Here's how the part is built. I have some questions about the finished solid (model axes, mm). Face numbers are marked on the shaded views. Coordinates: 2 decimals unless noted, no trailing zeros. Write each loop counter-clockwise with the first axis right and the second up, starting at its lowest first coordinate (ties: lowest second). Pieces come first, ordered by that corner, then holes.
(1) Imagine slicing it at C-C, the plane z = 0.75. List the corners of the cut face in (x, y) for me.
(2) Thinking about a two-plate mould opening in Y: for the marked faces 1, 2, 3 and 4, which applies, released by +Y, released by -Y, zero draft, split by the parting line, or undercut?
(3) Imagine slicing it at A-A, the plane y = -6.6. List the corners of the cut face in (x, z) for me, plus the area to 3 significant figures.
(4) For pin 1 Ø2.5 at (y, z) = (-11, 3) entering from -X; pin 2 Ø0.5 at (x, y) = (-6.5, 1) entering from -Z; pin 3 Ø3 at (x, z) = (-5, 5.5) entering from -Y, each with a flat end and sliding along its axis, tell me the tip position at first contact or that it passes through.
(5) Imagine slicing it at B-B, the plane x = 3. List the corners of the cut face in (y, z) for me.
(6) Please list where these lines run through material, in increasing order: probe 1 along X at (y, z) = (-6.5, 4); probe 2 along X at (y, z) = (-10.25, 4.25); probe 3 along Y at (x, z) = (-4.25, 4.25).
(7) Imagine slicing it at D-D, the plane y = -11.5. List the corners of the cut face in (x, z) for me, plus the area to 3 significant figures.
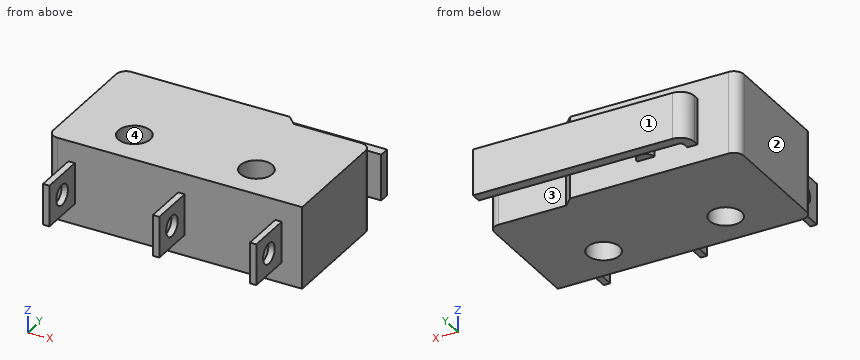
```python
from build123d import *

# Parameters (mm, degrees)
F0_W     = 0.5
F0_H     = 3.5
F0_R     = 1.25
F1_DEPTH = 6.4
F2_W     = 1.5
F2_H     = 1.4
F2_W_2   = 3.5
F2_H_2   = 1.6
F2_R     = 0.8
F3_DEPTH = 19.8
F4_R     = 0.762


with BuildPart() as f1:
    # F0 (on Top) → F1 (new body)
    with BuildSketch(Plane.XY):
        with Locations((4.1668843009, -11.25)):
            Rectangle(F0_W, F0_H)
        with Locations((-3.3831156991, -11.25)):
            Rectangle(F0_W, F0_H)
        with Locations((-11.9331156991, -11.25)):
            Rectangle(F0_W, F0_H)
        with BuildLine():
            Line((-10.6081156991, 0.7), (-9.8143656991, 0.7))
            Line((-9.8143656991, 0.7), (-9.8143656991, 1.101979753))
            ThreePointArc((-9.8143656991, 1.101979753), (-9.7252470071, 1.317131308), (-9.5100954521, 1.40625))
            Line((-9.5100954521, 1.40625), (6.0168843009, 1.40625))
            Line((6.0168843009, 1.40625), (6.0168843009, 2.2))
            Line((6.0168843009, 2.2), (-9.5100954521, 2.2))
            ThreePointArc((-9.5100954521, 2.2), (-10.2865130147, 1.8783973155), (-10.6081156991, 1.101979753))
            Line((-10.6081156991, 1.101979753), (-10.6081156991, 0.7))
        make_face()
        with BuildLine():
            Line((6.0168843009, 0), (0, 0))
            Line((0, 0), (-0.7, 0.7))
            Line((-0.7, 0.7), (-5.9126656991, 0.7))
            ThreePointArc((-5.9126656991, 0.7), (-6.5935156991, 1.38085), (-7.2743656991, 0.7))
            Line((-7.2743656991, 0.7), (-9.8143656991, 0.7))
            Line((-9.8143656991, 0.7), (-10.6081156991, 0.7))
            Line((-10.6081156991, 0.7), (-13.7831156991, 0.7))
            Line((-13.7831156991, 0.7), (-13.7831156991, -9.5))
            Line((-13.7831156991, -9.5), (-12.1831156991, -9.5))
            Line((-12.1831156991, -9.5), (-11.6831156991, -9.5))
            Line((-11.6831156991, -9.5), (-3.6331156991, -9.5))
            Line((-3.6331156991, -9.5), (-3.1331156991, -9.5))
            Line((-3.1331156991, -9.5), (3.9168843009, -9.5))
            Line((3.9168843009, -9.5), (4.4168843009, -9.5))
            Line((4.4168843009, -9.5), (6.0168843009, -9.5))
            Line((6.0168843009, -9.5), (6.0168843009, 0))
        make_face()
        with Locations((-8.6831156991, -6.6)):
            Circle(F0_R, mode=Mode.SUBTRACT)
        with Locations((0.8168843009, -6.6)):
            Circle(F0_R, mode=Mode.SUBTRACT)
    extrude(amount=F1_DEPTH)

    # F2 (on face) → F3 (cut, through all)
    with BuildSketch(Plane(origin=(-13.7831156991, 0, 0), x_dir=(0, -1, 0), z_dir=(-1, 0, 0))):
        with Locations((-1.45, 0.7)):
            Rectangle(F2_W, F2_H)
        with Locations((-1.45, 5.7)):
            Rectangle(F2_W, F2_H)
        with Locations((11.25, 0.8)):
            Rectangle(F2_W_2, F2_H_2)
        with Locations((11.25, 5.6)):
            Rectangle(F2_W_2, F2_H_2)
        with Locations((11.25, 3.2)):
            Circle(F2_R)
    extrude(amount=-F3_DEPTH, mode=Mode.SUBTRACT)

    # F4
    f4_edges = [f1.edges().sort_by_distance(p)[0] for p in [
        (-13.783116, -9.5, 3.2),
        (6.016884, 0, 3.2),
        (-13.783116, 0.7, 3.2),
    ]]
    fillet(f4_edges, radius=F4_R)


solid = f1.part
```
Recorded:
1. outline: (-13.78, -8.74) arc R0.76 ccw to (-13.02, -9.5) - (6.02, -9.5) - (6.02, -0.76) arc R0.76 ccw to (5.25, 0) - (0, 0) - (-0.7, 0.7) - (-13.02, 0.7) arc R0.76 ccw to (-13.78, -0.06) - close; hole circle Ø2.5 at (-8.68, -6.6); hole circle Ø2.5 at (0.82, -6.6)
2. face 1: released by +Y
2. face 2: zero draft
2. face 3: undercut
2. face 4: undercut
3. outline: (-13.78, 0) - (-9.93, 0) - (-9.93, 6.4) - (-13.78, 6.4) - close; (-7.43, 0) - (-0.43, 0) - (-0.43, 6.4) - (-7.43, 6.4) - close; (2.07, 0) - (6.02, 0) - (6.02, 6.4) - (2.07, 6.4) - close
3. area: 94.7 mm2
4. pin 1: stops at x = -12.18
4. pin 2: stops at z = 1.4
4. pin 3: stops at y = -9.5
5. outline: (-9.5, 0) - (0, 0) - (0, 6.4) - (-9.5, 6.4) - close; (1.41, 1.4) - (2.2, 1.4) - (2.2, 5) - (1.41, 5) - close
6. probe 1: x = -13.78 to -9.93, -7.44 to -0.43, 2.06 to 6.02
6. probe 2: x = -12.18 to -11.68, -3.63 to -3.13, 3.92 to 4.42
6. probe 3: y = -9.5 to 0.7, 1.41 to 2.2
7. outline: (-12.18, 1.6) - (-11.68, 1.6) - (-11.68, 2.44) - (-12.18, 2.44) - close; (-12.18, 3.96) - (-11.68, 3.96) - (-11.68, 4.8) - (-12.18, 4.8) - close; (-3.63, 1.6) - (-3.13, 1.6) - (-3.13, 2.44) - (-3.63, 2.44) - close; (-3.63, 3.96) - (-3.13, 3.96) - (-3.13, 4.8) - (-3.63, 4.8) - close; (3.92, 1.6) - (4.42, 1.6) - (4.42, 2.44) - (3.92, 2.44) - close; (3.92, 3.96) - (4.42, 3.96) - (4.42, 4.8) - (3.92, 4.8) - close
7. area: 2.52 mm2
